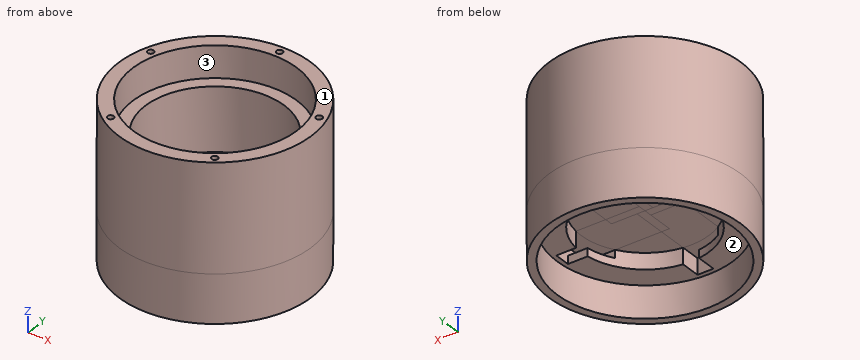
from build123d import *

# Parameters (mm, degrees)
SKETCH2_R           = 76.2
BOSS_EXTRUDE1_DEPTH = 85
SKETCH4_R           = 65
CUT_EXTRUDE2_DEPTH  = 25
SKETCH5_R           = 55
CUT_EXTRUDE3_DEPTH  = 50
SKETCH7_R           = 2.5
CUT_EXTRUDE4_DEPTH  = 20
CIRPATTERN1_COUNT   = 5
BOSS_EXTRUDE2_START = 38.1
SKETCH8_R           = 76.2
SKETCH8_R_2         = 50.8
BOSS_EXTRUDE2_DEPTH = 38.1
CUT_EXTRUDE5_DEPTH  = 66.04
CIRPATTERN2_COUNT   = 4
SKETCH12_R          = 69.85
CUT_EXTRUDE6_DEPTH  = 25.4


with BuildPart() as part:
    # Sketch2 → Boss-Extrude1 (new body)
    with BuildSketch(Plane(origin=(0, 0, 0), x_dir=(0, 1, 0), z_dir=(0, 0, 1))):
        with Locations(Location((0, 0, 0), (0, 0, 270))):
            Circle(SKETCH2_R)
    extrude(amount=BOSS_EXTRUDE1_DEPTH)

    # Sketch4 → Cut-Extrude2 (cut)
    with BuildSketch(Plane.XY.offset(85)):
        Circle(SKETCH4_R)
    extrude(amount=-CUT_EXTRUDE2_DEPTH, mode=Mode.SUBTRACT)

    # Sketch5 → Cut-Extrude3 (cut)
    with BuildSketch(Plane.XY.offset(60)):
        Circle(SKETCH5_R)
    extrude(amount=-CUT_EXTRUDE3_DEPTH, mode=Mode.SUBTRACT)

    # Sketch7 → Cut-Extrude4 (cut)
    with BuildSketch(Plane.XY.offset(85)):
        with Locations((0, 70.612)):
            Circle(SKETCH7_R)
    cut_extrude4 = extrude(amount=-CUT_EXTRUDE4_DEPTH, mode=Mode.SUBTRACT)

    # CirPattern1: Cut-Extrude4 ×5 about axis
    cirpattern1_axis = Axis((0, 0, 0), (0, 0, 1))
    for i in range(1, CIRPATTERN1_COUNT):
        add(cut_extrude4.rotate(cirpattern1_axis, i * 360 / CIRPATTERN1_COUNT), mode=Mode.SUBTRACT)

    # Sketch8 → Boss-Extrude2 (add)
    with BuildSketch(Plane(origin=(0, 0, 0), x_dir=(1, 0, 0), z_dir=(0, 0, -1)).offset(BOSS_EXTRUDE2_START)):
        with Locations(Location((0, 0, 0), (0, 0, 180))):
            Circle(SKETCH8_R)
        Circle(SKETCH8_R_2, mode=Mode.SUBTRACT)
    extrude(amount=-BOSS_EXTRUDE2_DEPTH)

    # Sketch10 → Cut-Extrude5 (cut)
    with BuildSketch(Plane(origin=(0, 0, 0), x_dir=(-1, 0, 0), z_dir=(0, 1, 0))):
        Polygon((-6.35, 0), (-6.35, -38.1), (6.35, -38.1), (6.35, -6.35), (26.709025115, -6.35), (26.709025115, 0), align=None)
    cut_extrude5 = extrude(amount=-CUT_EXTRUDE5_DEPTH, mode=Mode.SUBTRACT)

    # CirPattern2: Cut-Extrude5 ×4 about axis
    cirpattern2_axis = Axis((0, 0, 0), (0, 0, 1))
    for i in range(1, CIRPATTERN2_COUNT):
        add(cut_extrude5.rotate(cirpattern2_axis, i * 360 / CIRPATTERN2_COUNT), mode=Mode.SUBTRACT)

    # Sketch12 → Cut-Extrude6 (cut)
    with BuildSketch(Plane(origin=(0, 0, -38.1), x_dir=(1, 0, 0), z_dir=(0, 0, -1))):
        with Locations(Location((0, 0, 0), (0, 0, 180))):
            Circle(SKETCH12_R)
    extrude(amount=-CUT_EXTRUDE6_DEPTH, mode=Mode.SUBTRACT)


solid = part.part
Here's how the part is built. I have some questions about the finished solid (model axes, mm). Face numbers are marked on the shaded views. A direction names the side the tool comes from. Give positions to 0.01 mm unless a question says otherwise; leave off trailing zeros. Order: outer loops, then holes, each group sorted by start corner. A loop starts at its lowest first (then second) coordinate and runs counter-clockwise, first axis right, second up. Notation, with made-up numbers: (39, -21) -> (47, -21) arc R13 ccw to (47, -16) -> close; hole circle Ø8 at (-0.75, 17.25). An arc over 180 degrees is marked (long way). One line per item, written item: value. Start each with the question number.
1. I need wall thicknesses on probe 1 along Y at (x, z) = (0, 74); probe 2 along Y at (x, z) = (1, 59.5); probe 3 along Y at (x, z) = (-39.5, 68). Which ranges of each line are inside material? Lowest first, please. Write a range as from..to.
2. Will these pins go through, and if not, where does the flat tip stop? pin 1 Ø12 at (x, z) = (-56, 43.5) entering from -Y; pin 2 Ø5 at (x, y) = (33, 26.5) entering from +Z; pin 3 Ø5 at (y, z) = (-5.5, 34.5) entering from -X; pin 4 Ø10 at (x, y) = (28, -61) entering from -Z.
3. Imagine slicing it at B-B, the plane y = 48. List the corners of the cut face in (x, z) for me, plus the area to 3 significant figures.
4. Imagine slicing it at D-D, the plane z = 26. List the corners of the cut face in (x, y) for me, plus the area to 3 significant figures.
5. For the marked faces 1, 2 and 3, which set-ups out of +Z, -Z, +X, -X, +Y, -Y let a thin tool reach every point of the face, with its end or its side?
6. Imagine slicing it at C-C, the plane z = -30. List the corners of the cut face in (x, y) for me.
7. Imagine slicing it at A-A, the plane z = 70. List the corners of the cut face in (x, y) for me.
Values follow:
1. probe 1: y = -76.2..-65, 65..68.11, 73.11..76.2
1. probe 2: y = -76.19..-54.99, 54.99..76.19
1. probe 3: y = -65.16..-58.62, -55.63..-51.62, 51.62..65.16
2. pin 1: stops at y = -57.5
2. pin 2: stops at z = 10
2. pin 3: stops at x = -76.14
2. pin 4: stops at z = -38.1
3. outline: (-59.18, -38.1) -> (-50.74, -38.1) -> (-50.74, -12.7) -> (-16.63, -12.7) -> (-16.63, 0) -> (26.71, 0) -> (26.71, -6.35) -> (16.63, -6.35) -> (16.63, -12.7) -> (50.74, -12.7) -> (50.74, -38.1) -> (59.18, -38.1) -> (59.18, 85) -> (43.83, 85) -> (43.83, 60) -> (26.85, 60) -> (26.85, 10) -> (-26.85, 10) -> (-26.85, 60) -> (-43.83, 60) -> (-43.83, 85) -> (-59.18, 85) -> close
3. area: 6,630 mm2
4. outline: circle Ø152.4 at (0, 0); hole circle Ø110 at (0, 0)
4. area: 8,740 mm2
5. face 1: +Z, +X, -X, +Y, -Y
5. face 2: -Z
5. face 3: +Z
6. outline: circle Ø152.4 at (0, 0); hole circle Ø139.7 at (0, 0)
7. outline: circle Ø152.4 at (0, 0); hole circle Ø5 at (-67.16, 21.82); hole circle Ø130 at (0, 0); hole circle Ø5 at (-41.5, -57.13); hole circle Ø5 at (0, 70.61); hole circle Ø5 at (41.5, -57.13); hole circle Ø5 at (67.16, 21.82)
